Check sheet for the drawn part. Datum: minimum x, y, z corner. Units: mm. A direction names the side the tool comes from. Round coordinates to 2 decimals unless told otherwise and drop trailing zeros. Order: outer loops, then holes, each group sorted by start corner. A loop starts at its lowest first (then second) coordinate and runs counter-clockwise, first axis right, second up. Notation, with made-up numbers: M -13,-23.75 L 20,-23.75 A27 cw 20,-7.75 Z; hole C -30.75,33.25 d4. An arc over 180 degrees is marked long. Use one line per item in the form item = value. Start each with the question number.
Item 1: Cross-section at C-C on y = 4. Enter the section's corners in (x, z).
Item 2: Cross-section at A-A on z = 12. Enter the section's corners in (x, y) (3 decimals), then the cut area to 3 significant figures.
Item 3: Cross-section at B-B on x = 21. Enter the section's corners in (y, z), then the cut area to 3 significant figures.
Item 4: Go/stop test with flat-tipped pins: pin 1 Ø3 at (x, y) = (49, 12.5) entering from -Z; pin 2 Ø13 at (x, z) = (30, 7) entering from -Y. Record where each tip stops, or that it passes through.
Item 5: Cross-section at D-D on z = 4.5. Enter the section's corners in (x, y).
Item 6: Tool access check on the marked faces 1 and 2. Record the directions out of +Z, -Z, +X, -X, +Y, -Y that give a thin tool (end or side, any length) a straight path to the whole face; none if there is none.
Item 7: Thickness scan on probe 1 along X at (y, z) = (52.25, 12) (3 decimals); probe 2 along Z at (x, y) = (27, 14.5); probe 3 along Y at (x, z) = (36.5, 4.75). Record the ranges inside material, lowest first. Write a range as [from, to].
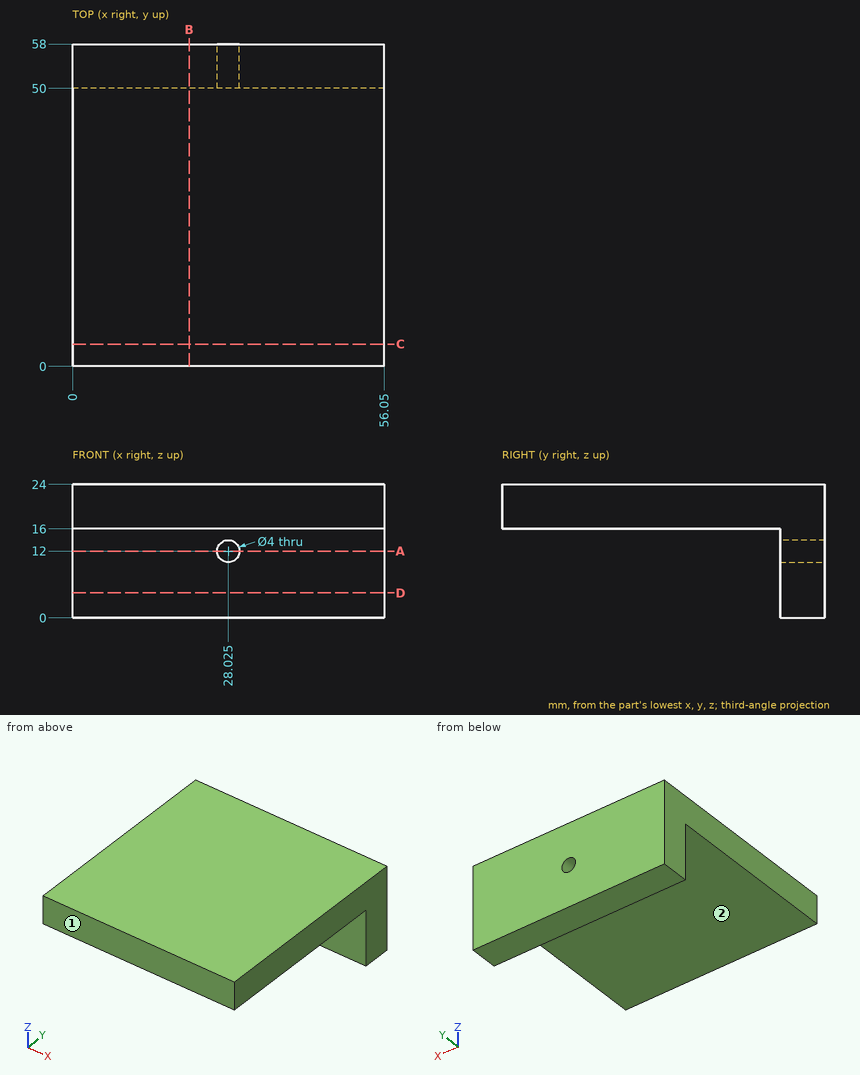
Output values:
q1.outline = M 0,16 L 56.05,16 L 56.05,24 L 0,24 Z
q2.outline = M 0,50 L 26.025,50 L 26.025,58 L 0,58 Z; M 30.025,50 L 56.05,50 L 56.05,58 L 30.025,58 Z
q2.area = 416 mm2
q3.outline = M 0,16 L 50,16 L 50,0 L 58,0 L 58,24 L 0,24 Z
q3.area = 592 mm2
q4.pin_1 = 16
q4.pin_2 = 50
q5.outline = M 0,50 L 56.05,50 L 56.05,58 L 0,58 Z
q6.face_1 = +Z, -Z, +X, -X, -Y
q6.face_2 = -Z, +X, -X, -Y
q7.probe_1 = [0, 26.025], [30.025, 56.05]
q7.probe_2 = [16, 24]
q7.probe_3 = [50, 58]
